from build123d import *

# Parameters (mm, degrees)
F0_R     = 40
F0_R_2   = 10.9
F1_DEPTH = 7
F2_R     = 5


# Not quite as in the source:
# - a fillet or chamfer that OpenCascade refuses, or shapes differently, is made with other operations: its cross-section is extruded or revolved along the edge and cut away or added


with BuildPart() as f1:
    # F0 (on Top) → F1 (new body)
    with BuildSketch(Plane.XY):
        Circle(F0_R)
        Circle(F0_R_2, mode=Mode.SUBTRACT)
    extrude(amount=F1_DEPTH)

    # F2
    f2_edges = [f1.edges().sort_by_distance(p)[0] for p in [
        (-40, 0, 7),
    ]]
    fillet(f2_edges, radius=F2_R)

    # F3: fillet of radius 5 on 1 edges, made by hand

    # F3_s1 → F3_t2 (revolve, cut)
    with BuildSketch(Plane.XZ):
        with BuildLine():
            ThreePointArc((40, 2), (38.2360679775, 0.527864045), (36, 0))
            Line((36, 0), (40, 0))
            Line((40, 0), (40, 2))
        make_face()
    revolve(axis=Axis((0, 0, 0), (0, 0, 1)), mode=Mode.SUBTRACT)


solid = f1.part
Could you check a few things on this model? Use its own coordinates, in mm. Coordinates: 2 decimals unless noted, no trailing zeros. Write each loop counter-clockwise with the first axis right and the second up, starting at its lowest first coordinate (ties: lowest second). Pieces come first, ordered by that corner, then holes. Notation, with made-up numbers: (-21, 53.5) - (5, 53.5) arc R23 cw to (5, 67.5) - close; hole circle Ø2 at (21.25, -7). An arc over 180 degrees is marked (long way). Put each result on its own line as item: value. Start each with the question number.
Q1. Please list where these lines run through material, in increasing order: L1, parallel to Y at x = -9, z = 4.5; L2, parallel to Y at x = 0, z = 4; L3, parallel to X at y = -30, z = 1.75.
Q2. I want a section at A-A on y = 0. Write out the boundary of the cut face in (x, z).
Q3. I want a section at C-C on z = 3.75. Write out the boundary of the cut face in (x, y), plus the area to 3 significant figures.
Checks:
1. L1: -38.29 to -6.15, 6.15 to 38.29
1. L2: -39.58 to -10.9, 10.9 to 39.58
1. L3: -26.15 to 26.15
2. outline: (-40, 2) arc R5 ccw to (-36, 0) - (-10.9, 0) - (-10.9, 7) - (-35, 7) arc R5 ccw to start; (10.9, 0) - (36, 0) arc R5 ccw to (40, 2) arc R5 ccw to (35, 7) - (10.9, 7) - close
3. outline: circle Ø79.37 at (0, 0); hole circle Ø21.8 at (0, 0)
3. area: 4,570 mm²
